```python
from build123d import *

# Parameters (mm, degrees)
SKETCH_1_W          = 44.75
SKETCH_1_H          = 50
EXTRUDE_1_DEPTH     = 30
SHELL_1_T           = 5
FILLET_1_R          = 5
SKETCH_2_R          = 0.75
CUT_EXTRUDE_1_DEPTH = 70.264438928
SKETCH_3_R          = 5
CUT_EXTRUDE_2_DEPTH = 70.264438928
EXTRUDE_2_DEPTH     = 30
CUT_EXTRUDE_3_DEPTH = 20
SKETCH_7_R          = 2.1
CUT_EXTRUDE_4_DEPTH = 159.731347329
SKETCH_8_W          = 18
SKETCH_8_H          = 45
CUT_EXTRUDE_5_DEPTH = 10
SKETCH_9_W          = 18
SKETCH_9_H          = 45
CUT_EXTRUDE_6_DEPTH = 10
FILLET_2_R          = 3
SKETCH_10_W         = 85.567589514
SKETCH_10_H         = 51.13951385
CUT_EXTRUDE_7_DEPTH = 122.018141743
CUT_EXTRUDE_8_DEPTH = 156.88457272
SKETCH_12_R         = 5
SKETCH_12_R_2       = 0.75
CUT_EXTRUDE_9_DEPTH = 154.138857117


with BuildPart() as part:
    # 草图1 → 凸台-拉伸1 (new body)
    with BuildSketch(Plane.XY):
        Rectangle(SKETCH_1_W, SKETCH_1_H)
    extrude(amount=EXTRUDE_1_DEPTH)

    # 抽壳1
    shell_1_openings = [part.faces().sort_by_distance(p)[0] for p in [
        (0, -25, 15),
        (0, 0, 0),
        (0, 0, 30),
    ]]
    offset(amount=SHELL_1_T, openings=shell_1_openings, kind=Kind.INTERSECTION)

    # 圆角1
    # the kernel refuses this fillet: 5 mm, written as the material it takes off along each edge
    with BuildSketch(Plane(origin=(-27.375, 30, -12.5), x_dir=(1, 0, 0), z_dir=(0, 0, 1)), Plane(origin=(-27.375, -25, 42.5), x_dir=(1, 0, 0), z_dir=(0, 0, -1)), Plane(origin=(27.375, -25, -12.5), x_dir=(-1, 0, 0), z_dir=(0, 0, 1)), Plane(origin=(27.375, 30, 42.5), x_dir=(-1, 0, 0), z_dir=(0, 0, -1))) as fillet_1_piece_1:
        with BuildLine():
            CenterArc((FILLET_1_R, -FILLET_1_R), FILLET_1_R, 90, 90)
            Line((0, -FILLET_1_R), (0, 0))
            Line((0, 0), (FILLET_1_R, 0))
        make_face()
    extrude(amount=55, mode=Mode.SUBTRACT)
    with BuildSketch(Plane(origin=(-27.375, -37.5, 30), x_dir=(1, 0, 0), z_dir=(0, 1, 0)), Plane(origin=(27.375, 42.5, 30), x_dir=(-1, 0, 0), z_dir=(0, -1, 0))) as fillet_1_piece_2:
        with BuildLine():
            CenterArc((FILLET_1_R, FILLET_1_R), FILLET_1_R, 180, 90)
            Line((0, FILLET_1_R), (0, 0))
            Line((0, 0), (FILLET_1_R, 0))
        make_face()
    extrude(amount=80, mode=Mode.SUBTRACT)
    with BuildSketch(Plane(origin=(-27.375, -37.5, 0), x_dir=(1, 0, 0), z_dir=(0, 1, 0)), Plane(origin=(27.375, 42.5, 0), x_dir=(-1, 0, 0), z_dir=(0, -1, 0))) as fillet_1_piece_3:
        with BuildLine():
            CenterArc((FILLET_1_R, -FILLET_1_R), FILLET_1_R, 90, 90)
            Line((0, -FILLET_1_R), (0, 0))
            Line((0, 0), (FILLET_1_R, 0))
        make_face()
    extrude(amount=80, mode=Mode.SUBTRACT)

    # 草图2 → 切除-拉伸1 (cut, through all)
    with BuildSketch(Plane.ZY.offset(27.375)):
        with Locations(Location((15, 7, 0), (0, 0, 270))):
            Circle(SKETCH_2_R)
        with Locations(Location((12, 7, 0), (0, 0, 270))):
            Circle(SKETCH_2_R)
        with Locations(Location((18, 7, 0), (0, 0, 270))):
            Circle(SKETCH_2_R)
        with Locations(Location((8, -3, 0), (0, 0, 90))):
            Circle(SKETCH_2_R)
        with Locations(Location((8, 0, 0), (0, 0, 90))):
            Circle(SKETCH_2_R)
        with Locations(Location((8, 3, 0), (0, 0, 90))):
            Circle(SKETCH_2_R)
        with Locations(Location((12, -7, 0), (0, 0, 90))):
            Circle(SKETCH_2_R)
        with Locations(Location((15, -7, 0), (0, 0, 90))):
            Circle(SKETCH_2_R)
        with Locations(Location((18, -7, 0), (0, 0, 90))):
            Circle(SKETCH_2_R)
        with Locations(Location((22, -3, 0), (0, 0, 270))):
            Circle(SKETCH_2_R)
        with Locations(Location((22, 0, 0), (0, 0, 270))):
            Circle(SKETCH_2_R)
        with Locations(Location((22, 3, 0), (0, 0, 270))):
            Circle(SKETCH_2_R)
    extrude(amount=-CUT_EXTRUDE_1_DEPTH, mode=Mode.SUBTRACT)

    # 草图3 → 切除-拉伸2 (cut, through all)
    with BuildSketch(Plane(origin=(27.375, 0, 0), x_dir=(0, 0, -1), z_dir=(1, 0, 0))):
        with Locations(Location((-15, 0, 0), (0, 0, 90))):
            Circle(SKETCH_3_R)
    extrude(amount=-CUT_EXTRUDE_2_DEPTH, mode=Mode.SUBTRACT)

    # 草图4 → 凸台-拉伸2 (add)
    with BuildSketch(Plane.XY.offset(30)):
        Polygon((0, 30), (-15, 30), (-15, 150), (15, 150), (15, 30), align=None)
    extrude(amount=-EXTRUDE_2_DEPTH)

    # 草图6 → 切除-拉伸3 (cut)
    with BuildSketch(Plane.XY.offset(30)):
        Polygon((-15, 99), (15, 99), (15, 141), (5, 141), (5, 150), (-15, 150), (-15, 141), align=None)
    extrude(amount=-CUT_EXTRUDE_3_DEPTH, mode=Mode.SUBTRACT)

    # 草图7 → 切除-拉伸4 (cut, through all)
    with BuildSketch(Plane(origin=(15, 0, 0), x_dir=(0, 0, -1), z_dir=(1, 0, 0))):
        with Locations((-24.925, 144.75)):
            Circle(SKETCH_7_R)
        with Locations((-15.075, 144.75)):
            Circle(SKETCH_7_R)
        with Locations(Location((-15.075, 95.25, 0), (0, 0, 180))):
            Circle(SKETCH_7_R)
        with Locations(Location((-24.925, 95.25, 0), (0, 0, 180))):
            Circle(SKETCH_7_R)
    extrude(amount=-CUT_EXTRUDE_4_DEPTH, mode=Mode.SUBTRACT)

    # 草图8 → 切除-拉伸5 (cut)
    with BuildSketch(Plane.XY.offset(30)):
        with Locations((0, 64.5)):
            Rectangle(SKETCH_8_W, SKETCH_8_H)
    extrude(amount=-CUT_EXTRUDE_5_DEPTH, mode=Mode.SUBTRACT)

    # 草图9 → 切除-拉伸6 (cut)
    with BuildSketch(Plane(origin=(0, 0, 0), x_dir=(-1, 0, 0), z_dir=(0, 0, -1))):
        with Locations((0, 65)):
            Rectangle(SKETCH_9_W, SKETCH_9_H)
    extrude(amount=-CUT_EXTRUDE_6_DEPTH, mode=Mode.SUBTRACT)

    # 圆角2
    fillet_2_edges = [part.edges().sort_by_distance(p)[0] for p in [
        (-15, 90, 0),
        (15, 90, 0),
        (15, 64.5, 30),
        (-15, 64.5, 30),
    ]]
    fillet(fillet_2_edges, radius=FILLET_2_R)

    # 草图10 → 切除-拉伸7 (cut, through all)
    with BuildSketch(Plane(origin=(0, 89, 0), x_dir=(1, 0, 0), z_dir=(0, 1, 0))):
        with Locations((0, -19.677859547)):
            Rectangle(SKETCH_10_W, SKETCH_10_H)
    extrude(amount=-CUT_EXTRUDE_7_DEPTH, mode=Mode.SUBTRACT)

    # 草图11 → 切除-拉伸8 (cut, through all)
    with BuildSketch(Plane(origin=(15, 0, 0), x_dir=(0, 0, -1), z_dir=(1, 0, 0))):
        Polygon((-10, 99), (-10, 141), (-5, 141), (-4.484921434, 99), align=None)
    extrude(amount=-CUT_EXTRUDE_8_DEPTH, mode=Mode.SUBTRACT)

    # 草图12 → 切除-拉伸9 (cut, through all)
    with BuildSketch(Plane(origin=(0, -0.040106419, 3.270315816), x_dir=(1, 0, 0), z_dir=(0, -0.012262853244216906, 0.9999248083882663))):
        with Locations(Location((0, 120.133486449, 0), (0, 0, 270))):
            Circle(SKETCH_12_R)
        with Locations(Location((7.084353343, 120.133486449, 0), (0, 0, 270))):
            Circle(SKETCH_12_R_2)
        with Locations(Location((7.084353343, 117.133486449, 0), (0, 0, 270))):
            Circle(SKETCH_12_R_2)
        with Locations(Location((3.077588855, 127.014955444, 0), (0, 0, 270))):
            Circle(SKETCH_12_R_2)
        with Locations(Location((-2.922031664, 127.082435984, 0), (0, 0, 270))):
            Circle(SKETCH_12_R_2)
        with Locations(Location((-7.084353343, 123.133486449, 0), (0, 0, 270))):
            Circle(SKETCH_12_R_2)
        with Locations(Location((-7.084353343, 117.133486449, 0), (0, 0, 270))):
            Circle(SKETCH_12_R_2)
        with Locations(Location((-3, 113.217839792, 0), (0, 0, 270))):
            Circle(SKETCH_12_R_2)
        with Locations(Location((0, 113.217839792, 0), (0, 0, 270))):
            Circle(SKETCH_12_R_2)
        with Locations(Location((3, 113.217839792, 0), (0, 0, 270))):
            Circle(SKETCH_12_R_2)
        with Locations(Location((7.084353343, 123.133486449, 0), (0, 0, 270))):
            Circle(SKETCH_12_R_2)
        with Locations(Location((0.077778595, 127.048695714, 0), (0, 0, 270))):
            Circle(SKETCH_12_R_2)
        with Locations(Location((-7.084353343, 120.133486449, 0), (0, 0, 270))):
            Circle(SKETCH_12_R_2)
    extrude(amount=-CUT_EXTRUDE_9_DEPTH, mode=Mode.SUBTRACT)


solid = part.part
```
Input: part model. Units: mm. Frame: model coordinates. Give positions to 0.01 mm unless a question says otherwise; leave off trailing zeros. Order: outer loops, then holes, each group sorted by start corner. A loop starts at its lowest first (then second) coordinate and runs counter-clockwise, first axis right, second up. Notation, with made-up numbers: (14, 87) - (46, 87) arc R19 cw to (46, 124) - close; hole circle Ø6 at (-10.75, 79). An arc over 180 degrees is marked (long way). Use a Markdown table: item, result.
(1) Section query D-D (z = 25). Output: boundary loops of the cut face in (x, y), then the cut area to 3 significant figures.
Computed values:
| item | result |
|---|---|
| outline | (-15, 89) - (15, 89) - (15, 93.15) - (-15, 93.15) - close; (-15, 97.35) - (15, 97.35) - (15, 99) - (-15, 99) - close; (5, 141) - (15, 141) - (15, 142.65) - (5, 142.65) - close; (5, 146.85) - (15, 146.85) - (15, 150) - (5, 150) - close |
| area | 222 mm2 |
(2) Line query: line 1 (Z direction, x = 7.5, y = 144.75) (3 decimals); line 2 (Y direction, x = 11, z = 25); line 3 (Y direction, x = 13, z = 5.5). Output: solid intervals per line, ascending. Write a range as from..to.
Computed values:
| item | result |
|---|---|
| line 1 | z = 0..12.975, 17.175..22.825, 27.025..30 |
| line 2 | y = 89..93.15, 97.35..99, 141..142.65, 146.85..150 |
| line 3 | y = 89..99, 141..150 |
(3) Pin query (flat end, axial travel): pin 1 (2 mm diameter, centred on x = 3.5, z = 19, fed in from +Y); pin 2 (1 mm diameter, centred on x = 5, y = 116.5, fed in from +Z); pin 3 (10 mm diameter, centred on x = -5.5, y = 146.5, fed in from +Z). Return the tip coordinate at first contact, or that it passes through.
Computed values:
| item | result |
|---|---|
| pin 1 | stops at y = 99 |
| pin 2 | stops at z = 4.71 |
| pin 3 | stops at z = 10 |
(4) Section query B-B (x = 11). Output: boundary loops of the cut face in (y, z) (3 decimals).
Computed values:
| item | result |
|---|---|
| outline | (89, 0) - (150, 0) - (150, 30) - (141, 30) - (141, 5) - (99, 4.485) - (99, 30) - (89, 30) - close; hole circle Ø4.2 at (95.25, 15.075); hole circle Ø4.2 at (95.25, 24.925); hole circle Ø4.2 at (144.75, 15.075); hole circle Ø4.2 at (144.75, 24.925) |
(5) Section query C-C (x = -10). Output: boundary loops of the cut face in (y, z) (3 decimals).
Computed values:
| item | result |
|---|---|
| outline | (89, 0) - (150, 0) - (150, 10) - (141, 10) - (141, 5) - (99, 4.485) - (99, 30) - (89, 30) - close; hole circle Ø4.2 at (95.25, 15.075); hole circle Ø4.2 at (95.25, 24.925) |
(6) Section query A-A (y = 144.75). Output: boundary loops of the cut face in (x, z) (3 decimals), then the cut area to 3 significant figures.
Computed values:
| item | result |
|---|---|
| outline | (-15, 3) arc R3 ccw to (-12, 0) - (12, 0) arc R3 ccw to (15, 3) - (15, 12.975) - (5, 12.975) - (5, 10) - (-15, 10) - close; (5, 17.175) - (15, 17.175) - (15, 22.825) - (5, 22.825) - close; (5, 27.025) - (15, 27.025) - (15, 30) - (5, 30) - close |
| area | 412 mm2 |
(7) Draft query along X for faces 1 (the cylindrical face through (7.591, 117.666, 2.389)), 2 (the flat face through (10, 146, 30)), 3 (the flat face through (15, 117.38, 4.56)), 4 (the cylindrical face through (-14.1, 92, 29.14)). Return one class per face: released by +X, released by -X, zero draft, split by the parting line, or undercut.
Computed values:
| item | result |
|---|---|
| face 1 | undercut |
| face 2 | zero draft |
| face 3 | released by +X |
| face 4 | released by -X |
